Read the model definition and answer for the solid it produces. Units are mm, in the model's axes. Face numbers are marked on the shaded views. A direction names the side the tool comes from. Coordinates: 2 decimals unless noted, no trailing zeros. Loops run counter-clockwise (first coordinate to the right, second up) from the corner with the lowest first, then second, coordinate; pieces in that order, holes last. Notation, with made-up numbers: M -34,-29 L 15,-29 A17 cw 15,-15 Z; hole C 67,42.25 d8. An arc over 180 degrees is marked long. One line per item, written item: value. Start each with the question number.
```python
from build123d import *

# Parameters (mm, degrees)
BOX002_W          = 20
BOX002_H          = 3
BOX002_DEPTH      = 100
ARRAY001_COUNT    = 8
CYLINDER005_R     = 9
CYLINDER005_DEPTH = 20
CYLINDER004_R     = 15
CYLINDER004_DEPTH = 20


with BuildPart() as almenas:
    # Box002 → Box002 (new body)
    with BuildSketch(Plane(origin=(7, 0, 50), x_dir=(1, 0, 0), z_dir=(0, 0, 1))):
        with Locations((10, 1.5)):
            Rectangle(BOX002_W, BOX002_H)
    extrude(amount=BOX002_DEPTH)

    # Array001: Almenas ×8 about axis
    array001_axis = Axis((0, 0, 0), (0, 0, 1))


with BuildPart() as almenas_1:
    add(almenas.part)
    for i in range(1, ARRAY001_COUNT):
        add(almenas.part.rotate(array001_axis, i * 360 / ARRAY001_COUNT))


with BuildPart() as cilindro003:
    # Cylinder005 → Cylinder005 (new body)
    with BuildSketch(Plane.XY.offset(40)):
        Circle(CYLINDER005_R)
    extrude(amount=CYLINDER005_DEPTH)


with BuildPart() as parte_superior:
    # Cylinder004 → Cylinder004 (new body)
    with BuildSketch(Plane.XY.offset(40)):
        Circle(CYLINDER004_R)
    extrude(amount=CYLINDER004_DEPTH)

    # Cut002: cut Cilindro003
    add(cilindro003.part, mode=Mode.SUBTRACT)

    # Cut003: cut Almenas
    add(almenas_1.part, mode=Mode.SUBTRACT)


solid = parte_superior.part
```
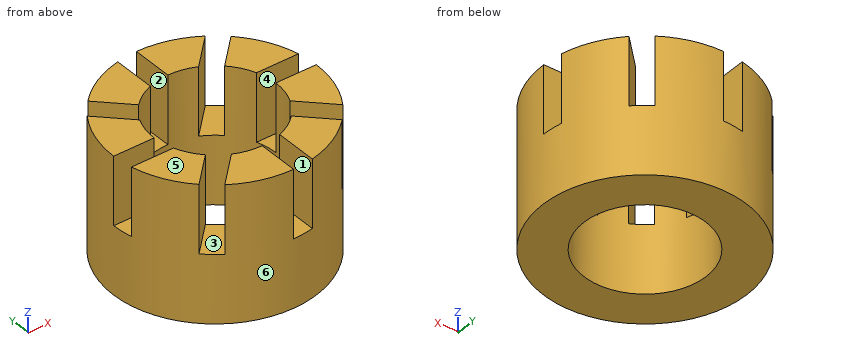
1) Consider line 1 along Y through (x, z) = (-8, 57); line 2 along Y through (x, z) = (3, 49.5); line 3 along X through (y, z) = (11.75, 58.25). Determine where each line is inside the solid, lowest interval first.
2) For a pull along Y with two mould halves and no side action, classify the marked faces 4, 5 and 6 as released by +Y, released by -Y, zero draft, split by the parting line, or undercut.
3) A tool of negligible diameter and unlimited length cuts with its end or side. For the marked faces 1, 2 and 3, from which of +Z, -Z, +X, -X, +Y, -Y can it reach the whole face along a straight path? Write none if from no direction.
4) Section A-A (z = 52.25) is taken. Count the separate pieces of the cut face and the enclosed holes in it, then the cut area to 3 significant figures.
5) Section D-D (z = 46) is taken. Determine the outline of the cut face in (x, y), then the cut area to 3 significant figures.
6) Flat-ended cylindrical pins translate along their axes: pin 1 (7 mm diameter, centred on x = 7.5, y = 10, fed in from +Z); pin 2 (1.8 mm diameter, centred on y = -12.5, z = 55, fed in from +X); pin 3 (5 mm diameter, centred on x = -11.5, z = 53, fed in from +Y); pin 4 (2.5 mm diameter, centred on x = -1.5, y = 10.5, fed in from +Z). Find the tip coordinate at first contact, or state that the pin passes through.
7) Section B-B (y = -5) is taken. Determine the outline of the cut face in (x, z).
8) Section C-C (x = 4.75) is taken. Determine the outline of the cut face in (y, z).
Results found:
1. line 1: y = -12.69 to -12.24, -8 to -4.12, 8 to 12.69
1. line 2: y = -14.7 to -8.49, 8.49 to 14.7
1. line 3: x = -9.32 to -3, 0 to 7.51
2. face 4: undercut
2. face 5: zero draft
2. face 6: split by the parting line
3. face 1: +Z, -Y
3. face 2: +Z, +Y
3. face 3: +Z
4. separate pieces: 8
4. enclosed holes: 0
4. area: 307 mm²
5. outline: C 0,0 d30; hole C 0,0 d18
5. area: 452 mm²
6. pin 1: stops at z = 60
6. pin 2: stops at x = 9.51
6. pin 3: stops at y = 12
6. pin 4: stops at z = 50
7. outline: M -14.14,40 L -7.48,40 L -7.48,60 L -14.14,60 Z; M 7.48,40 L 14.14,40 L 14.14,60 L 9.24,60 L 9.24,50 L 7.48,50 Z
8. outline: M -14.23,40 L -7.64,40 L -7.64,60 L -14.23,60 Z; M 7.64,40 L 14.23,40 L 14.23,60 L 8.99,60 L 8.99,50 L 7.64,50 Z
